CAD build for the part. Positions are in the model's coordinates, mm. A direction names the side the tool comes from. Round coordinates to 2 decimals unless told otherwise and drop trailing zeros. Loops run counter-clockwise (first coordinate to the right, second up) from the corner with the lowest first, then second, coordinate; pieces in that order, holes last. Notation, with made-up numbers: (38, 48.5) -> (70, 48.5) arc R12 ccw to (70, 61.5) -> close; hole circle Ø3 at (4, 43.25). An arc over 180 degrees is marked (long way). Answer as CSV lines item,"result".
```python
from build123d import *

# Parameters (mm, degrees)
F0_R     = 15
F0_R_2   = 10
F1_DEPTH = 25
F2_DEPTH = 50
F3_R     = 30
F3_R_2   = 10
F4_DEPTH = 25


# Not quite as in the source:
# - a feature names something its author has since deleted; it is built from what else it names


with BuildPart() as f1:
    # F0 (on Front) → F1 (new body)
    with BuildSketch(Plane.XZ):
        with BuildLine():
            ThreePointArc((6.25, -29.3417364858), (23.3184476327, -18.8745860882), (30, 0))
            ThreePointArc((30, 0), (23.3184476327, 18.8745860882), (6.25, 29.3417364858))
            ThreePointArc((6.25, 29.3417364858), (-30, 0), (6.25, -29.3417364858))
        make_face()
        Circle(F0_R, mode=Mode.SUBTRACT)
        with BuildLine():
            ThreePointArc((6.25, 29.3417364858), (23.3184476327, 18.8745860882), (30, 0))
            ThreePointArc((30, 0), (23.3184476327, -18.8745860882), (6.25, -29.3417364858))
            Line((6.25, -29.3417364858), (63.6458333333, -17.11601295))
            ThreePointArc((63.6458333333, -17.11601295), (42.5, 0), (63.6458333333, 17.11601295))
            Line((63.6458333333, 17.11601295), (6.25, 29.3417364858))
        make_face()
        with BuildLine():
            ThreePointArc((77.5, 0), (73.6024277858, 11.0101752181), (63.6458333333, 17.11601295))
            ThreePointArc((63.6458333333, 17.11601295), (42.5, 0), (63.6458333333, -17.11601295))
            ThreePointArc((63.6458333333, -17.11601295), (73.6024277858, -11.0101752181), (77.5, 0))
        make_face()
        with Locations((60, 0)):
            Circle(F0_R_2, mode=Mode.SUBTRACT)
    extrude(amount=F1_DEPTH)

    # F0 (on Front) → F2 (join)
    with BuildSketch(Plane.XZ):
        with BuildLine():
            ThreePointArc((6.25, -29.3417364858), (23.3184476327, -18.8745860882), (30, 0))
            ThreePointArc((30, 0), (23.3184476327, 18.8745860882), (6.25, 29.3417364858))
            ThreePointArc((6.25, 29.3417364858), (-30, 0), (6.25, -29.3417364858))
        make_face()
        Circle(F0_R, mode=Mode.SUBTRACT)
    extrude(amount=F2_DEPTH)

    # F3 (on face) → F4 (join)
    with BuildSketch(Plane(origin=(0, 0, 0), x_dir=(-1, 0, 0), z_dir=(0, 1, 0))):
        with Locations((-60, 0)):
            Circle(F3_R)
        with Locations((-60, 0)):
            Circle(F3_R_2, mode=Mode.SUBTRACT)
    extrude(amount=F4_DEPTH)


solid = f1.part
```
Q1. Probe L1, parallel to X at y = 21.5, z = 0.5; L2, parallel to Z at x = 60, y = 5; L3, parallel to Y at x = -4, z = -21. List the from-to ranges inside material, lowest first. Write a range as [from, to].
Results:
L1,"[30, 50.01], [69.99, 90]"
L2,"[-30, -10], [10, 30]"
L3,"[-50, 0]"
Q2. Two-plate mould, pull along Z, no slides. Class faces 1 (the flat face through (35.35, -12.325, 23.143)), 2 (the flat face through (76.4, 0, 7.1)), 3 (the cylindrical face through (-14.985, -24.65, 0.66)), 4 (the flat face through (34.546, -12.325, -23.314)): pulls with the +Z half, pulls with the -Z half, needs draft (parallel to the pull), parting line crosses it, or undercut.
Results:
face 1,"pulls with the +Z half"
face 2,"needs draft"
face 3,"undercut"
face 4,"pulls with the -Z half"
Q3. Tool access for faces 5 (the flat face through (47, 25, 0)), 6 (the cylindrical face through (-30, -30, 0)), 7 (the cylindrical face through (89.97, 12.32, 1.32)): list every direction of +Z, -Z, +X, -X, +Y, -Y with a clear straight run to the whole face (end or side of a thin tool).
Results:
face 5,"+Z, -Z, +X, -X, +Y"
face 6,"-Y"
face 7,"+Y"
Q4. Slice it at A-A, the plane y = -4. Give the cut face in (x, z), and give its area (3 significant figures).
Results:
outline,"(6.25, -29.34) -> (63.65, -17.12) arc R17.5 ccw to (63.65, 17.12) -> (6.25, 29.34) arc R30 ccw (long way) to start; hole circle Ø30 at (0, 0); hole circle Ø20 at (60, 0)"
area,"3,790 mm2"
Q5. Slice it at D-D, the plane z = -3. Give the cut face in (x, y), and give its area (3 significant figures).
Results:
outline,"(-29.85, -50) -> (-14.7, -50) -> (-14.7, 0) -> (-29.85, 0) -> close; (14.7, -50) -> (29.85, -50) -> (29.85, -25) -> (50.46, -25) -> (50.46, 25) -> (30.15, 25) -> (30.15, 0) -> (14.7, 0) -> close; (69.54, -25) -> (77.24, -25) -> (77.24, 0) -> (89.85, 0) -> (89.85, 25) -> (69.54, 25) -> close"
area,"3,240 mm2"
Q6. Drop flat-ended pins along their axis: pin 1 Ø18 at (x, z) = (9, -8.5) entering from +Y; pin 2 Ø5 at (x, z) = (46, -21) entering from -Y; pin 3 Ø3 at (y, z) = (-14.5, -8) entering from -X; pin 4 Ø18 at (x, z) = (60, 0) entering from -Y. Give the stop position or say it passes through.
Results:
pin 1,"y = 0"
pin 2,"y = -25"
pin 3,"x = -29.29"
pin 4,"through"
Q7. Slice it at C-C, the plane z = 25. Give the cut face in (x, y).
Results:
outline,"(-16.58, -50) -> (16.58, -50) -> (16.58, -25) -> (26.63, -25) -> (26.63, 0) -> (-16.58, 0) -> close; (43.42, 0) -> (76.58, 0) -> (76.58, 25) -> (43.42, 25) -> close"
Q8. Slice it at B-B, the plane x = 0. Give the cut face in (y, z), and give its area (3 significant figures).
Results:
outline,"(-50, -30) -> (0, -30) -> (0, -15) -> (-50, -15) -> close; (-50, 15) -> (0, 15) -> (0, 30) -> (-50, 30) -> close"
area,"1,500 mm2"
